```python
from build123d import *
from build123d import SkipClean  # not in build123d's __all__

# Parameters (mm, degrees)
F1_DEPTH = 6.35
F2_DEPTH = 6.35
F3_SIZE2 = 6.34999
F3_SIZE  = 6.34999
F4_DEPTH = 0.0254
F5_DEPTH = 0.0254
F7_DEPTH = 25.4
F8_DEPTH = 0.0254
F9_DEPTH = 0.0254


# Not quite as in the source:
# - a fillet or chamfer is up to 0.001 mm smaller than in the source, because OpenCascade refuses the exact size
# - ends of sketch curves that miss each other by under 0.0002 mm in the source are joined


with BuildPart() as f1:
    # F0 (on Front) → F1 (new body)
    with BuildSketch(Plane.XZ):
        Polygon((-17.139416188, 28.1973872334), (-27.9807504267, 3.4191238228), (0, -37.7674587071), (27.964355424, 3.4191238228), (17.08493568, 28.1973872334), (17.08493568, 469.1244959831), (0, 506.7884922028), (-17.139416188, 469.1244959831), align=None)
    extrude(amount=F1_DEPTH)

    # F2 (add): a face of the model
    f2_faces = [f1.faces().sort_by_distance(p)[0] for p in [
        (-0.0248835797, 0, 225.9211420486),
    ]]
    extrude(f2_faces, amount=F2_DEPTH)

    # F3 (size 6.35 and 6.35 in the source; OpenCascade refuses exactly that, so slightly less here)
    f3_edges = [f1.edges().sort_by_distance(p)[0] for p in [
        (-22.560083, -6.35, 15.808256),
        (-13.990375, -6.35, -17.174167),
        (13.982178, -6.35, -17.174167),
        (22.524646, -6.35, 15.808256),
        (17.084936, -6.35, 248.660942),
        (8.542468, -6.35, 487.956494),
        (-8.569708, -6.35, 487.956494),
        (-17.139416, -6.35, 248.660942),
        (-22.560083, 6.35, 15.808256),
        (-13.990375, 6.35, -17.174167),
        (13.982178, 6.35, -17.174167),
        (22.524646, 6.35, 15.808256),
        (17.084936, 6.35, 248.660942),
        (8.542468, 6.35, 487.956494),
        (-8.569708, 6.35, 487.956494),
        (-17.139416, 6.35, 248.660942),
    ]]
    chamfer(f3_edges, length=F3_SIZE, length2=F3_SIZE2)

    # F4 (add): a face of the model
    f4_faces = [f1.faces().sort_by_distance(p)[0] for p in [
        (-0.0252861091, -6.35, 223.0026633937),
    ]]
    extrude(f4_faces, amount=F4_DEPTH)

    # F5 (add): a face of the model
    f5_faces = [f1.faces().sort_by_distance(p)[0] for p in [
        (-0.0252861091, 6.35, 223.0026633937),
    ]]
    extrude(f5_faces, amount=F5_DEPTH)

    # F6 (on face) → F7 (cut)
    with BuildSketch(Plane.XZ.offset(6.3754)):
        Polygon((10.73493568, 467.7515936734), (10.73493568, 99.0661755204), (32.7086560428, 99.0661755204), (32.7086560428, 505.495429039), (10.73493568, 505.495429039), (10.73493568, 501.6054906496), (19.4450523704, 491.0283088684), (13.1097852611, 474.0980863571), (20.738528953, 474.0980863571), (20.738528953, 467.7515928086), align=None)
        Polygon((32.7086560428, 99.0661755204), (10.73493568, 99.0661755204), (10.73493568, 29.554810375), (20.738528953, 31.6301956773), (21.6034320424, 29.554810375), (32.7086560428, 29.554810375), align=None)
        Polygon((20.738528953, 31.6301956773), (10.73493568, 29.554810375), (21.6034320424, 29.554810375), align=None)
        Polygon((21.6034320424, 29.554810375), (10.73493568, 29.554810375), (10.73493568, 26.8647358603), (20.738530435, 4.0811948515), (27.3526439581, -1.5923568075), (32.2193913162, 4.0811982268), align=None)
        Polygon((-0.0092029974, 491.4372314137), (10.73494568, 467.7515949707), (10.73493568, 474.0980863571), (10.73493568, 501.6054906496), (0, 514.6415233612), (-11.796230803, 486.6769015789), (-10.789416188, 486.6769015789), (-10.789416188, 467.7476089999), align=None)
        Polygon((13.1097852611, 474.0980863571), (10.73493568, 467.7515928086), (20.738528953, 467.7515928086), (20.738528953, 474.0980863571), align=None)
        Polygon((10.73493568, 474.0980863571), (10.73493568, 467.7515936734), (13.1097852611, 474.0980863571), align=None)
        Polygon((10.73493568, 501.6054906496), (10.73493568, 474.0980863571), (13.1097852611, 474.0980863571), (19.4450523704, 491.0283088684), align=None)
        Polygon((27.3526439581, -1.5923568075), (20.738528953, 4.0811982268), (24.6255261009, -4.7715753101), align=None)
        Polygon((24.6255261009, -4.7715753101), (20.738530435, 4.0811948515), (-0.0015394217, -26.4652965043), (0, -41.624262929), (29.7397422671, -3.639997893), (27.3526439581, -1.5923568075), align=None)
        Polygon((-16.2565966219, 476.1029779911), (-10.789416188, 467.7476075543), (-10.789416188, 486.6769015789), (-11.796230803, 486.6769015789), align=None)
        Polygon((-10.789416188, 26.8690092904), (-10.789416188, 467.7476089999), (-16.2565966219, 476.1029779911), (-11.796230803, 486.6769015789), (-21.7237770557, 486.6769015789), (-21.7237770557, 26.8690092904), (-20.8278130876, 26.8690092904), (-18.3457657695, 33.1129990518), align=None)
        Polygon((0, -41.624262929), (-0.0015394241, -26.4652787056), (-20.7574730934, 4.0866529625), (-30.316057774, 2.9998017031), align=None)
        Polygon((-20.8278130876, 26.8690092904), (-10.789416188, 26.8690092904), (-18.3457657695, 33.1129990518), align=None)
        Polygon((-20.7574730934, 4.0866529625), (-10.789416188, 26.8690092904), (-20.8278130876, 26.8690092904), (-30.316057774, 2.9998017031), align=None)
    with SkipClean():  # cleaning this boolean's faces spoils the solid; the shape is the same uncleaned
        extrude(amount=-F7_DEPTH, mode=Mode.SUBTRACT)

    # F8 (cut): a face of the model
    f8_faces = [f1.faces().sort_by_distance(p)[0] for p in [
        (-0.0252861091, -6.3754, 223.0026633937),
    ]]
    extrude(f8_faces, amount=-F8_DEPTH, mode=Mode.SUBTRACT)

    # F9 (cut): a face of the model
    f9_faces = [f1.faces().sort_by_distance(p)[0] for p in [
        (-0.0252864299, 6.3754, 223.0026587516),
    ]]
    extrude(f9_faces, amount=-F9_DEPTH, mode=Mode.SUBTRACT)


solid = f1.part
```
Geometry: final body of the model. Coordinates: model frame, mm. A direction names the side the tool comes from. Coordinates: 2 decimals unless noted, no trailing zeros. Order: outer loops, then holes, each group sorted by start corner. A loop starts at its lowest first (then second) coordinate and runs counter-clockwise, first axis right, second up. Notation, with made-up numbers: (-24.5, -2) -> (-8.5, -2) arc R27 cw to (-8.5, 28) -> close; hole circle Ø4 at (50, -7.5). An arc over 180 degrees is marked (long way). Write item = value, one per line.
(1) Line query: line 1 (X direction, y = -3, z = 316.5); line 2 (Z direction, x = 7.5, y = -5.5); line 3 (X direction, y = 5.75, z = 12). Output: solid intervals per line, ascending.
Solved:
line_1 = -10.79 to 10.73
line_2 = -15.42 to 474.88
line_3 = -17.3 to 17.26
(2) Cut plane A-A on y = -1.75. Return loops of the section in (x, z).
Solved:
outline = (-20.76, 4.09) -> (0, -26.47) -> (20.74, 4.08) -> (10.73, 26.86) -> (10.73, 467.75) -> (-0.01, 491.44) -> (-10.79, 467.75) -> (-10.79, 26.87) -> close
(3) Cut plane C-C on x = 16. Return loops of the section in (y, z), plus the area to 3 significant figures.
Solved:
outline = (-6.35, -2.9) -> (6.35, -2.9) -> (6.35, 14.87) -> (-6.35, 14.87) -> close
area = 226 mm²
(4) Cut plane B-B on z = 279. Return loops of the section in (x, y), plus the area to 3 significant figures.
Solved:
outline = (-10.79, -6.35) -> (10.73, -6.35) -> (10.73, 6.35) -> (-10.79, 6.35) -> close
area = 273 mm²
(5) Pin query (flat end, axial travel): pin 1 Ø1 at (x, y) = (11, -4.5) entering from +Z; pin 2 Ø3 at (x, y) = (14.5, 4) entering from -Z; pin 3 Ø3 at (y, z) = (-1.5, 185.5) entering from -X. Return the tip coordinate at first contact, or that it passes through.
Solved:
pin_1 = 468.27
pin_2 = -7.32
pin_3 = -10.79
(6) Access query for faces 1 (the flat face through (10.735, 0, 250)), 2 (the flat face through (-10.234, -0.089, -11.403)), 3 (the flat face through (-10.789, 0, 244)). Directions: +Z, -Z, +X, -X, +Y, -Y. A direction counts if a zero-diameter tool reaches every point of the face in a straight line with its end or side. Return the directions, or none.
Solved:
face_1 = +Z, +X, +Y, -Y
face_2 = -Z, -X, +Y, -Y
face_3 = +Z, -X, +Y, -Y
